For this review, use the dimensioned drawing (mm, ordinates from the lowest corner) and the shaded views. A direction names the side the tool comes from. Coordinates: 2 decimals unless noted, no trailing zeros. Loops run counter-clockwise (first coordinate to the right, second up) from the corner with the lowest first, then second, coordinate; pieces in that order, holes last. Notation, with made-up numbers: M 47,2.25 L 84,2.25 A19 cw 84,18.25 Z; hole C -30.75,34.5 d9. An arc over 180 degrees is marked long. Write each question's results on one line, items separated by ' | '. Start each with the question number.
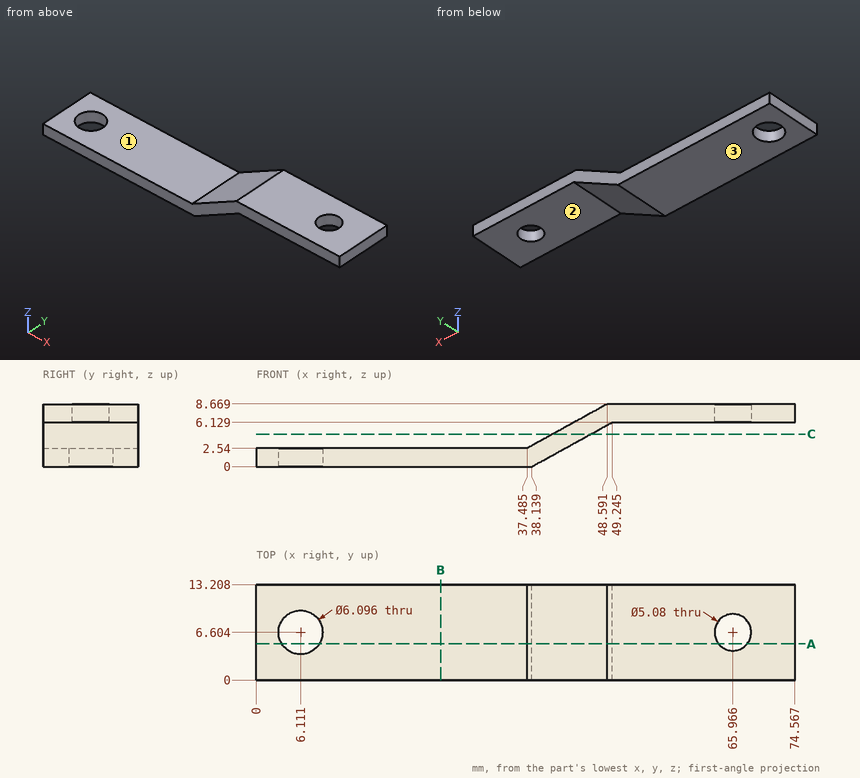
Q1. Take a section at C-C, the plane z = 4.5. Give the boundary of the cut face in (x, y).
Q2. To check wall thickness, follow line 1 along Z through (x, y) = (64, 11); line 2 along X through (y, z) = (4.75, 6.5) (1 decimal); line 3 along X through (y, z) = (7, 6.5) (1 decimal). State the ranges of each line that lie inside material, in increasing order.
Q3. Take a section at A-A, the plane y = 5. Give the boundary of the cut face in (x, z) (1 decimal), then the cut area to 3 significant figures.
Q4. For the marked faces 1, 2 and 3, list the 3-axis set-ups (+Z, -Z, +X, -X, +Y, -Y) from which the entire face can be reached by the end or side of a thin tool; tool diameter is ignored.
Q5. Take a section at B-B, the plane x = 25.5. Give the boundary of the cut face in (y, z).
Q6. Insertion check: P1, Ø4, axis at x = 65.97, y = 6.6, coming from the -Z side; P2, Ø4, axis at x = 10, y = 6.5, coming from the +Z side; P3, Ø4, axis at x = 57, y = 9, coming from the -Z side; P4, Ø4, axis at y = 9, z = 5, coming from the -X side. Each pin has a flat end and moves straight along its axis. Give the tip position at first contact, or say it passes through.
Results:
1) outline: M 41.04,0 L 46.29,0 L 46.29,13.21 L 41.04,13.21 Z
2) line 1: 6.13 to 8.67 | line 2: 44.7 to 64.2, 67.7 to 74.6 | line 3: 44.7 to 63.5, 68.5 to 74.6
3) outline: M 0,0 L 3.5,0 L 3.5,2.5 L 0,2.5 Z; M 8.7,0 L 38.1,0 L 49.2,6.1 L 64,6.1 L 64,8.7 L 48.6,8.7 L 37.5,2.5 L 8.7,2.5 Z; M 67.9,6.1 L 74.6,6.1 L 74.6,8.7 L 67.9,8.7 Z | area: 170 mm^2
4) face 1: +Z, -X, +Y, -Y | face 2: -Z, +X, +Y, -Y | face 3: -Z, +X, -X, +Y, -Y
5) outline: M 0,0 L 13.21,0 L 13.21,2.54 L 0,2.54 Z
6) P1: through | P2: z = 2.54 | P3: z = 6.13 | P4: x = 38.32
